from build123d import *

# Parameters (mm, degrees)
F1_DEPTH = 2.4


with BuildPart() as f1:
    # F0 (on Front) → F1 (new body)
    with BuildSketch(Plane.XZ):
        with BuildLine():
            Line((-10.5, 18.9), (-10.5, 10.712143))
            ThreePointArc((-10.5, 10.712143), (-15, 0), (-10.5, -10.712143))
            Line((-10.5, -10.712143), (-10.5, -18.9))
            Line((-10.5, -18.9), (0, -18.9))
            Line((0, -18.9), (0, -15.8))
            Line((0, -15.8), (10.5, -15.8))
            Line((10.5, -15.8), (10.5, -10.712143))
            ThreePointArc((10.5, -10.712143), (15, 0), (10.5, 10.712143))
            Line((10.5, 10.712143), (10.5, 15.8))
            Line((10.5, 15.8), (0, 15.8))
            Line((0, 15.8), (0, 18.9))
            Line((0, 18.9), (-10.5, 18.9))
        make_face()
    extrude(amount=F1_DEPTH)


solid = f1.part
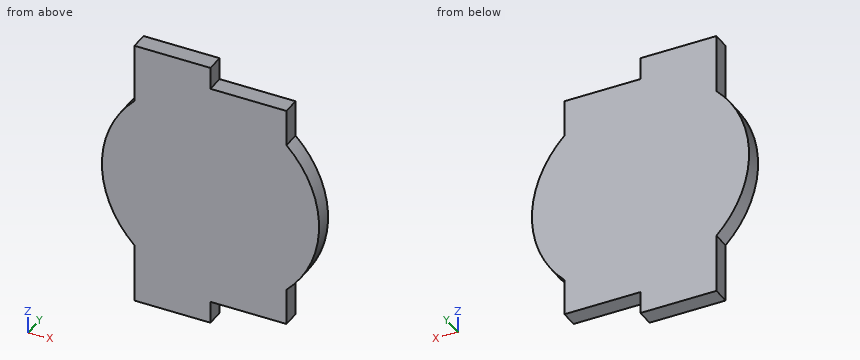
Check sheet for the modelled part. Datum: model origin and axes. Units: mm. Give positions to 0.01 mm unless a question says otherwise; leave off trailing zeros. Loops run counter-clockwise (first coordinate to the right, second up) from the corner with the lowest first, then second, coordinate; pieces in that order, holes last. Notation, with made-up numbers: M 41.5,5 L 79.5,5 A17 ccw 79.5,27 Z; hole C 88,61 d3. An arc over 180 degrees is marked long. Answer as a JSON object with one key per item and string values. Group by question number.
Q1. Material ranges on line 1 along X through (y, z) = (-1.2, 14); line 2 along Z through (x, y) = (5.25, -1.2); line 3 along X through (y, z) = (-0.45, -0.5), recorded low to high. Write a range as [from, to].
Q2. Go/stop test with flat-tipped pins: P1, Ø0.7, axis at y = -1.5, z = -15.5, coming from the -X side; P2, Ø1.2, axis at x = 8, y = -1, coming from the +Z side; P3, Ø0.7, axis at y = -1.5, z = -18, coming from the +X side. Record where each tip stops, or that it passes through.
Q3. Cross-section at A-A on y = -1.95. Record the cut outline in (x, z), then the cut area to 3 significant figures.
Q4. Cross-section at C-C on x = 2.75. Record the cut outline in (y, z), then the cut area to 3 significant figures.
Q5. Cross-section at B-B on z = -12.5. Record the cut outline in (x, y), then the cut area to 3 significant figures.
Evaluation:
{
 "1": {"line 1": "x = [-10.5, 10.5]", "line 2": "z = [-15.8, 15.8]", "line 3": "x = [-14.99, 14.99]"},
 "2": {"P1": "stops at x = -10.5", "P2": "stops at z = 15.8", "P3": "stops at x = 0"},
 "3": {"outline": "M -10.5,-18.9 L 0,-18.9 L 0,-15.8 L 10.5,-15.8 L 10.5,-10.71 A15 ccw 10.5,10.71 L 10.5,15.8 L 0,15.8 L 0,18.9 L -10.5,18.9 L -10.5,10.71 A15 ccw -10.5,-10.71 Z", "area": "862 mm2"},
 "4": {"outline": "M -2.4,-15.8 L 0,-15.8 L 0,15.8 L -2.4,15.8 Z", "area": "75.8 mm2"},
 "5": {"outline": "M -10.5,-2.4 L 10.5,-2.4 L 10.5,0 L -10.5,0 Z", "area": "50.4 mm2"}
}
